Part model, mm, in its own coordinate system. A direction names the side the tool comes from. Round coordinates to 2 decimals unless told otherwise and drop trailing zeros. Write each loop counter-clockwise with the first axis right and the second up, starting at its lowest first coordinate (ties: lowest second). Pieces come first, ordered by that corner, then holes. Notation, with made-up numbers: (36.25, 30) -> (54.25, 30) arc R19 cw to (54.25, 52) -> close; hole circle Ø11 at (69, -12.75). An arc over 180 degrees is marked (long way). Return JSON: item names as keys, results as strings. Group by question number.
(1) Saw through at A-A (x = 0). List the corners of the cut face in (y, z) (3 decimals), plus the area to 3 significant figures.
(2) Saw through at D-D (x = 18). List the corners of the cut face in (y, z).
(3) Mould opens along Y. For faces 1 (the cylindrical face through (-3.108, -13.994, 8.08)), 2 (the cylindrical face through (23.05, 7.26, 8.08)), 3 (the flat face through (20, -12, 16.39)) say: +Y half, -Y half, draft (parallel to the pull), parting line (faces both ways), or undercut.
(4) Saw through at C-C (z = 13.5). List the corners of the cut face in (x, y) (3 decimals).
(5) Drill centre lines: L1, parallel to Y at x = 0, z = 8.25 (3 decimals); L2, parallel to Y at x = 6.5, z = 5.5; L3, parallel to X at y = 4.5, z = 11.25. Where is each one in solid material? Low to high. Write a range as from..to.
(6) Tool access for faces 4 (the flat face through (15, -5, 1)), 5 (the flat face through (10.4, -10.4, 0)): list every direction of +Z, -Z, +X, -X, +Y, -Y with a clear straight run to the whole face (end or side of a thin tool).
(7) Drop flat-ended pins along their axis: pin 1 Ø17 at (x, y) = (0, 0) entering from +Z; pin 2 Ø4 at (x, z) = (-17.5, 7) entering from -Y; pin 3 Ø1.5 at (y, z) = (-13.5, 4.5) entering from +X. Give the stop position or say it passes through.
from build123d import *

# Parameters (mm, degrees)
F0_R     = 24.165
F0_R_2   = 14.335
F1_DEPTH = 0.1
F2_DEPTH = 16.29
F3_T     = -1


with BuildPart() as f1:
    # F0 (on Top) → F1 (new body)
    with BuildSketch(Plane.XY):
        Circle(F0_R)
        Circle(F0_R_2, mode=Mode.SUBTRACT)
    extrude(amount=F1_DEPTH)

    # F2 (add): a face of the model
    f2_faces = [f1.faces().sort_by_distance(p)[0] for p in [
        (-23.4815105853, 0, 0.1),
    ]]
    extrude(f2_faces, amount=F2_DEPTH)

    # F3
    f3_openings = [f1.faces().sort_by_distance(p)[0] for p in [
        (-23.481511, 0, 16.39),
    ]]
    offset(amount=F3_T, openings=f3_openings)


solid = f1.part
Computed values:
{
 "1": {"outline": "(-24.165, 0) -> (-14.335, 0) -> (-14.335, 16.39) -> (-15.335, 16.39) -> (-15.335, 1) -> (-23.165, 1) -> (-23.165, 16.39) -> (-24.165, 16.39) -> close; (14.335, 0) -> (24.165, 0) -> (24.165, 16.39) -> (23.165, 16.39) -> (23.165, 1) -> (15.335, 1) -> (15.335, 16.39) -> (14.335, 16.39) -> close", "area": "81.2 mm2"},
 "2": {"outline": "(-16.12, 0) -> (16.12, 0) -> (16.12, 16.39) -> (14.58, 16.39) -> (14.58, 1) -> (-14.58, 1) -> (-14.58, 16.39) -> (-16.12, 16.39) -> close"},
 "3": {"face 1": "undercut", "face 2": "parting line", "face 3": "draft"},
 "4": {"outline": "circle Ø48.33 at (0, 0); circle Ø30.67 at (0, 0); hole circle Ø46.33 at (0, 0); hole circle Ø28.67 at (0, 0)"},
 "5": {"L1": "-24.165..-23.165, -15.335..-14.335, 14.335..15.335, 23.165..24.165", "L2": "-23.27..-22.23, -13.89..-12.78, 12.78..13.89, 22.23..23.27", "L3": "-23.74..-22.72, -14.66..-13.61, 13.61..14.66, 22.72..23.74"},
 "6": {"face 4": "+Z", "face 5": "-Z, +X, -X, +Y, -Y"},
 "7": {"pin 1": "through", "pin 2": "y = -18.54", "pin 3": "x = 20.53"}
}
